Geometry check sheet. Reference: the model listing, model coordinates, mm. Face numbers are marked on the shaded views. A direction names the side the tool comes from. Give positions to 0.01 mm unless a question says otherwise; leave off trailing zeros. Write each loop counter-clockwise with the first axis right and the second up, starting at its lowest first coordinate (ties: lowest second). Pieces come first, ordered by that corner, then holes. Notation, with made-up numbers: M -39.75,-8.75 L 2.25,-8.75 A18 ccw 2.25,11.25 Z; hole C 54.5,15.5 d1. An arc over 180 degrees is marked long. Use one line per item in the form item = value. Start each with the question number.
```python
from build123d import *

# Parameters (mm, degrees)
SKETCH1_W                       = 80
SKETCH1_H                       = 122
BOSS_EXTRUDE1_DEPTH             = 3
BOSS_EXTRUDE2_DEPTH             = 8
SKETCH4_R                       = 6.45
CUT_EXTRUDE1_DEPTH              = 6
CHAMFER1_SIZE                   = 2
FILLET1_R                       = 2
F_2_5MM_DOWEL_HOLE1_D           = 2.5
F_2_5MM_DOWEL_HOLE1_DEPTH       = 5
F_2_5MM_DOWEL_HOLE1_CSINK_D     = 2.55
F_2_5MM_DOWEL_HOLE1_CSINK_ANGLE = 90
F_2_5MM_DOWEL_HOLE1_TIP         = 0.751075774
F_2_5MM_DOWEL_HOLE2_D           = 2.5
F_2_5MM_DOWEL_HOLE2_DEPTH       = 5
F_2_5MM_DOWEL_HOLE2_CSINK_D     = 2.55
F_2_5MM_DOWEL_HOLE2_CSINK_ANGLE = 90
F_2_5MM_DOWEL_HOLE2_TIP         = 0.751075774


with BuildPart() as part:
    # Sketch1 → Boss-Extrude1 (new body)
    with BuildSketch(Plane(origin=(0, 0, 0), x_dir=(1, 0, 0), z_dir=(0, 1, 0))):
        Rectangle(SKETCH1_W, SKETCH1_H)
    extrude(amount=BOSS_EXTRUDE1_DEPTH)

    # Sketch3 → Boss-Extrude2 (add)
    with BuildSketch(Plane(origin=(6, 0, 0), x_dir=(0, 0, -1), z_dir=(1, 0, 0))):
        with BuildLine():
            Line((-61, 0), (-61, -10))
            ThreePointArc((-61, -10), (-50.36, -20.64), (-39.72, -10))
            Line((-39.72, -10), (-39.72, 0))
            Line((-39.72, 0), (-61, 0))
        make_face()
        with BuildLine():
            Line((61, 0), (61, -10))
            ThreePointArc((61, -10), (50.36, -20.64), (39.72, -10))
            Line((39.72, -10), (39.72, 0))
            Line((39.72, 0), (61, 0))
        make_face()
    extrude(amount=BOSS_EXTRUDE2_DEPTH)

    # Sketch4 → Cut-Extrude1 (cut)
    with BuildSketch(Plane.ZY.offset(-6)):
        with Locations((-50.36, -10)):
            Circle(SKETCH4_R)
        with Locations((50.36, -10)):
            Circle(SKETCH4_R)
    extrude(amount=-CUT_EXTRUDE1_DEPTH, mode=Mode.SUBTRACT)

    # Chamfer1
    chamfer1_edges = [part.edges().sort_by_distance(p)[0] for p in [
        (6, 0, 50.36),
        (10, 0, 39.72),
        (14, 0, 50.36),
        (6, 0, -50.36),
        (10, 0, -39.72),
        (14, 0, -50.36),
    ]]
    chamfer(chamfer1_edges, length=CHAMFER1_SIZE)

    # Fillet1
    fillet1_edges = [part.edges().sort_by_distance(p)[0] for p in [
        (40, 1.5, 61),
        (-40, 1.5, 61),
        (-40, 1.5, -61),
        (40, 1.5, -61),
    ]]
    fillet(fillet1_edges, radius=FILLET1_R)

    # Ø2.5mm Dowel Hole1
    with Locations(Plane(origin=(0, 3, 0), x_dir=(1, 0, 0), z_dir=(0, 1, 0))):
        with Locations((-30, 51), (-30, -51), (30, -51), (30, 51)):
            CounterSinkHole(F_2_5MM_DOWEL_HOLE1_D / 2, F_2_5MM_DOWEL_HOLE1_CSINK_D / 2, depth=F_2_5MM_DOWEL_HOLE1_DEPTH, counter_sink_angle=F_2_5MM_DOWEL_HOLE1_CSINK_ANGLE)
            with Locations((0, 0, -(F_2_5MM_DOWEL_HOLE1_DEPTH + F_2_5MM_DOWEL_HOLE1_TIP / 2))):  # 118° drill point
                Cone(0, F_2_5MM_DOWEL_HOLE1_D / 2, F_2_5MM_DOWEL_HOLE1_TIP, mode=Mode.SUBTRACT)

    # Ø2.5mm Dowel Hole2
    with Locations(Plane.ZY.offset(-12)):
        with Locations((-50.36, -10), (50.36, -10)):
            CounterSinkHole(F_2_5MM_DOWEL_HOLE2_D / 2, F_2_5MM_DOWEL_HOLE2_CSINK_D / 2, depth=F_2_5MM_DOWEL_HOLE2_DEPTH, counter_sink_angle=F_2_5MM_DOWEL_HOLE2_CSINK_ANGLE)
            with Locations((0, 0, -(F_2_5MM_DOWEL_HOLE2_DEPTH + F_2_5MM_DOWEL_HOLE2_TIP / 2))):  # 118° drill point
                Cone(0, F_2_5MM_DOWEL_HOLE2_D / 2, F_2_5MM_DOWEL_HOLE2_TIP, mode=Mode.SUBTRACT)


solid = part.part
```
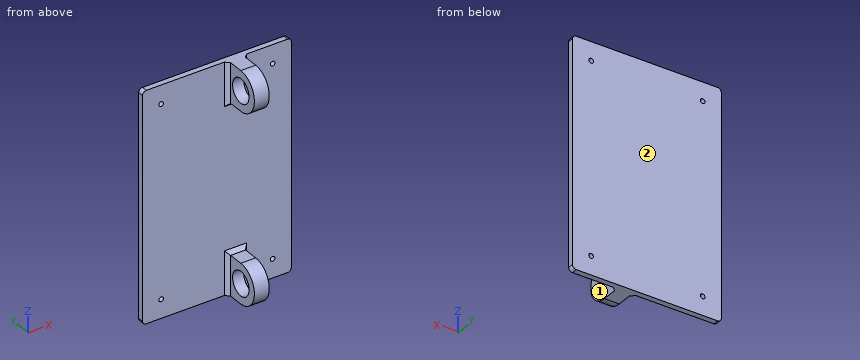
(1) Sectioned sample at A-A, the plane x = 30. Record the boundary of the cut face in (y, z) (3 decimals), plus the area to 3 significant figures.
(2) Thickness scan on probe 1 along X at (y, z) = (2.35, 51); probe 2 along Z at (x, y) = (-30, 1.5); probe 3 along Z at (x, y) = (12.7, -10). Record the ranges inside material, lowest first. Write a range as [from, to].
(3) Sectioned sample at C-C, the plane z = -41.5. Record the boundary of the cut face in (x, y), plus the area to 3 significant figures.
(4) Sectioned sample at B-B, the plane y = -15. Record the boundary of the cut face in (x, z).
(5) Tool access check on the marked faces 1 and 2. Record the directions out of +Z, -Z, +X, -X, +Y, -Y that give a thin tool (end or side, any length) a straight path to the whole face; none if there is none.
(6) Sectioned sample at D-D, the plane x = -12. Record the boundary of the cut face in (y, z), plus the area to 3 significant figures.
(7) Depth check by flat-ended pin: pin 1 (10 mm diameter, centred on y = -7.5, z = 48.5, fed in from -X); pin 2 (4 mm diameter, centred on y = -7.5, z = -48.5, fed in from -X); pin 3 (2 mm diameter, centred on x = 30, z = -51, fed in from +Y); pin 4 (4 mm diameter, centred on x = 30, z = 51, fed in from -Y). Enter the tip coordinate at first touch or a pass-through.
Numbers:
q1.outline = M 0,-61 L 3,-61 L 3,-52.275 L 2.975,-52.25 L 0,-52.25 Z; M 0,-49.75 L 2.975,-49.75 L 3,-49.725 L 3,49.725 L 2.975,49.75 L 0,49.75 Z; M 0,52.25 L 2.975,52.25 L 3,52.275 L 3,61 L 0,61 Z
q1.area = 351 mm2
q2.probe_1 = [-40, -31.25], [-28.75, 28.75], [31.25, 40]
q2.probe_2 = [-61, -52.25], [-49.75, 49.75], [52.25, 61]
q2.probe_3 = [-61, -51.61], [-49.11, -39.72], [39.72, 49.11], [51.61, 61]
q3.outline = M -40,0 L 4,0 L 6,-2 L 6,-15.89 L 14,-15.89 L 14,-2 L 16,0 L 40,0 L 40,3 L -40,3 Z
q3.area = 371 mm2
q4.outline = M 6,-59.75 L 14,-59.75 L 14,-40.97 L 6,-40.97 L 6,-46.29 L 12,-46.29 L 12,-54.43 L 6,-54.43 Z; M 6,40.97 L 14,40.97 L 14,59.75 L 6,59.75 L 6,54.43 L 12,54.43 L 12,46.29 L 6,46.29 Z
q5.face_1 = +Z, -Z, +X, -Y
q5.face_2 = +Z, -Z, +X, -X, +Y
q6.outline = M 0,-61 L 3,-61 L 3,61 L 0,61 Z
q6.area = 366 mm2
q7.pin_1 = 6
q7.pin_2 = 12
q7.pin_3 = through
q7.pin_4 = 0
